```python
from build123d import *

# Parameters (mm, degrees)
SKETCH009_R        = 8.5
SKETCH009_R_2      = 2.5
PAD012_DEPTH       = 5.5
SKETCH006_R        = 1.7
SKETCH006_R_2      = 2.6
PAD005_DEPTH       = 15
SKETCH024_R        = 1.7
PAD013_DEPTH       = 3
SKETCH014_R        = 2
SKETCH014_R_2      = 1.2
POCKET011002_DEPTH = 28.351
SKETCH017_R        = 2.6
POCKET011003_DEPTH = 4.5
POCKET011004_DEPTH = 6


with BuildPart() as roller_copy:
    # Sketch009 → Pad012 (new body)
    with BuildSketch(Plane(origin=(7.8, 21.15, 52.75), x_dir=(1, 0, 0), z_dir=(0, 0, 1))):
        Circle(SKETCH009_R)
        Circle(SKETCH009_R_2, mode=Mode.SUBTRACT)
    extrude(amount=PAD012_DEPTH)


with BuildPart() as tensioner001:
    # Sketch006 → Pad005 (new body)
    with BuildSketch(Plane.XY.offset(48)):
        with BuildLine():
            ThreePointArc((0.3, 21.15), (7.088015, 13.683871), (15.164821, 19.732461))
            ThreePointArc((19.022004, 25.646185), (16.51278, 23.068036), (15.164821, 19.732461))
            Line((34.156005, 36.112383), (19.022004, 25.646185))
            ThreePointArc((37, 37), (35.510355, 36.77294), (34.156005, 36.112383))
            Line((37, 37), (62, 37))
            ThreePointArc((62, 37), (64.5, 39.5), (62, 42))
            Line((0.3, 42), (62, 42))
            Line((0.3, 21.15), (0.3, 42))
        make_face()
        with Locations((5.65, 36.65)):
            Circle(SKETCH006_R, mode=Mode.SUBTRACT)
        with Locations((7.8, 21.15)):
            Circle(SKETCH006_R_2, mode=Mode.SUBTRACT)
    extrude(amount=PAD005_DEPTH)

    # Sketch024 → Pad013 (new body)
    with BuildSketch(Plane(origin=(0, 0, 48), x_dir=(1, 0, 0), z_dir=(0, 0, -1))):
        with BuildLine():
            Line((0.3, -42), (10.899992, -42))
            Line((10.899992, -42), (10.899992, -36.659185))
            ThreePointArc((10.899992, -36.659185), (9.365563, -32.940945), (5.650018, -31.4))
            Line((5.650018, -31.4), (0.3, -31.4))
            Line((0.3, -31.4), (0.3, -42))
        make_face()
        with Locations((5.65, -36.65)):
            Circle(SKETCH024_R, mode=Mode.SUBTRACT)
    extrude(amount=PAD013_DEPTH)

    # Sketch014 → Pocket011002 (cut, through all)
    with BuildSketch(Plane(origin=(0, 42, 48), x_dir=(-1, 0, 0), z_dir=(0, 1, 0))):
        with Locations((-40, 7.5)):
            Circle(SKETCH014_R)
        with Locations((-16.7, 7.5)):
            Circle(SKETCH014_R_2)
    extrude(amount=-POCKET011002_DEPTH, mode=Mode.SUBTRACT)

    # Sketch017 → Pocket011003 (cut)
    with BuildSketch(Plane(origin=(0, 42, 48), x_dir=(-1, 0, 0), z_dir=(0, 1, 0))):
        with Locations((-16.7, 7.5)):
            Circle(SKETCH017_R)
    extrude(amount=-POCKET011003_DEPTH, mode=Mode.SUBTRACT)

    # Sketch025 → Pocket011004 (cut)
    with BuildSketch(Plane.XY.offset(63)):
        with BuildLine():
            Line((-0.494617, 43), (10.932914, 43))
            Line((10.932914, 36.653394), (10.932914, 43))
            ThreePointArc((5.582914, 31.303394), (9.365935, 32.870373), (10.932914, 36.653394))
            Line((-0.494617, 31.303394), (5.582914, 31.303394))
            Line((-0.494617, 31.303394), (-0.494617, 43))
        make_face()
    extrude(amount=-POCKET011004_DEPTH, mode=Mode.SUBTRACT)

    # Cut: cut roller_copy
    add(roller_copy.part, mode=Mode.SUBTRACT)


solid = tensioner001.part
```
Read the model definition and answer for the solid it produces. Units are mm, in the model's axes. A direction names the side the tool comes from. Give positions to 0.01 mm unless a question says otherwise; leave off trailing zeros. Write each loop counter-clockwise with the first axis right and the second up, starting at its lowest first coordinate (ties: lowest second). Pieces come first, ordered by that corner, then holes. Notation, with made-up numbers: (49, -36) -> (64, -36) arc R27 ccw to (64, -15) -> close; hole circle Ø9 at (-26, 23.5). An arc over 180 degrees is marked (long way). Answer in a Markdown table with one row per item.
1) Section D-D on z = 50 is taken. Give the vertices of the cut face in (x, y), plus the area to 3 significant figures.
Results list:
| item | result |
|---|---|
| outline | (0.3, 21.15) arc R7.5 ccw to (15.16, 19.73) arc R9.34 cw to (19.02, 25.65) -> (34.16, 36.11) arc R5 cw to (37, 37) -> (62, 37) arc R2.5 ccw to (62, 42) -> (0.3, 42) -> close; hole circle Ø3.4 at (5.65, 36.65); hole circle Ø5.2 at (7.8, 21.15) |
| area | 757 mm^2 |
2) Determine the mould class of faces 1 (the flat face through (4, 38, 45)), 2 (the cylindrical face through (18.763, 39.782, 53.918)), 3 (the cylindrical face through (7.24, 18.61, 50.34)) for opening direction Z: released by +Z, released by -Z, zero draft, split by the parting line, or undercut.
Results list:
| item | result |
|---|---|
| face 1 | released by -Z |
| face 2 | undercut |
| face 3 | zero draft |
3) Section C-C on y = 39.5 is taken. Give the vertices of the cut face in (x, z).
Results list:
| item | result |
|---|---|
| outline | (0.3, 45) -> (10.9, 45) -> (10.9, 48) -> (64.5, 48) -> (64.5, 63) -> (10.93, 63) -> (10.93, 57) -> (0.3, 57) -> close; hole circle Ø5.2 at (16.7, 55.5); hole circle Ø4 at (40, 55.5) |
4) A tool of negligible diameter and unlimited length cuts with its end or side. For faces 4 (the flat face through (25, 31, 48)), 5 (the cylindrical face through (9.33, 29.51, 55.46)), 6 (the flat face through (7, 38, 57)), 7 (the flat face through (16, 37.5, 54)), from which of +Z, -Z, +X, -X, +Y, -Y can it reach the whole face along a straight path? Write none if from no direction.
Results list:
| item | result |
|---|---|
| face 4 | -Z, +X, -Y |
| face 5 | -Y |
| face 6 | +Z, -X, +Y |
| face 7 | +Y |
5) Each of these flat-tipped pins is pushed along its axis until it touches: pin 1 Ø3.5 at (x, z) = (2.5, 46) entering from -Y; pin 2 Ø3 at (x, z) = (16.7, 55.5) entering from +Y; pin 3 Ø0.9 at (y, z) = (40, 47) entering from +X; pin 4 Ø3 at (x, y) = (7.8, 21.15) entering from -Z. Where does it stop, or does it pass through?
Results list:
| item | result |
|---|---|
| pin 1 | y = 31.4 |
| pin 2 | y = 37.5 |
| pin 3 | x = 10.9 |
| pin 4 | through |
6) Straight lines are drawn through the part: line 1 (Y direction, x = 7.8, z = 51.5); line 2 (Z direction, x = 12, y = 24.75); line 3 (Z direction, x = 16.7, y = 32.5). For each, find the intervals that lie inside material, in ascending order. Write a range as [from, to].
Results list:
| item | result |
|---|---|
| line 1 | [13.65, 18.55], [23.75, 42] |
| line 2 | [48, 52.75], [58.25, 63] |
| line 3 | [48, 54.3], [56.7, 63] |
7) Section B-B on x = 40 is taken. Give the vertices of the cut face in (y, z), plus the area to 3 significant figures.
Results list:
| item | result |
|---|---|
| outline | (37, 48) -> (42, 48) -> (42, 53.5) -> (37, 53.5) -> close; (37, 57.5) -> (42, 57.5) -> (42, 63) -> (37, 63) -> close |
| area | 55.0 mm^2 |
8) Section A-A on z = 55.5 is taken. Give the vertices of the cut face in (x, y).
Results list:
| item | result |
|---|---|
| outline | (0.3, 25.15) arc R8.5 cw to (15.5, 24.75) -> (15.5, 37.5) -> (14.1, 37.5) -> (14.1, 42) -> (0.3, 42) -> close; (17.9, 24.73) arc R9.34 cw to (19.02, 25.65) -> (34.16, 36.11) arc R5 cw to (37, 37) -> (38, 37) -> (38, 42) -> (19.3, 42) -> (19.3, 37.5) -> (17.9, 37.5) -> close; (42, 37) -> (62, 37) arc R2.5 ccw to (62, 42) -> (42, 42) -> close; hole circle Ø3.4 at (5.65, 36.65) |
